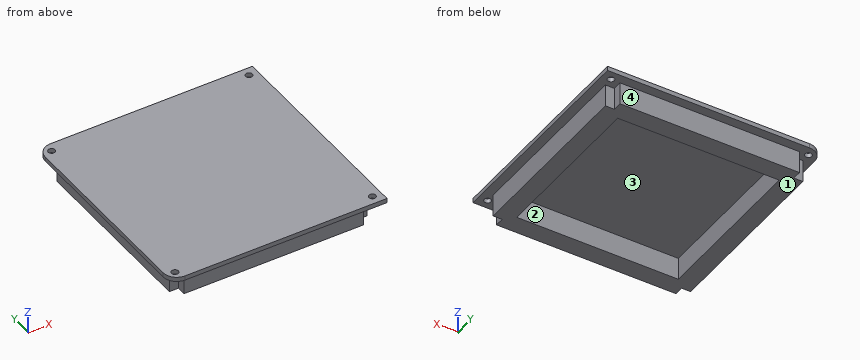
from build123d import *

# Parameters (mm, degrees)
F0_W     = 48
F0_H     = 48
F1_DEPTH = 1
F2_W     = 2
F2_H     = 2
F3_DEPTH = 5
F5_D     = 1.5
F6_R     = 3


with BuildPart() as f1:
    # F0 (on Top) → F1 (new body)
    with BuildSketch(Plane.XY):
        with Locations((-0.8524587825, -1.0040983325)):
            Rectangle(F0_W, F0_H)
        Polygon((19.1475412175, 18.9959016675), (21.1475412175, 18.9959016675), (21.1475412175, -21.0040983325), (19.1475412175, -21.0040983325), (19.1475412175, -23.0040983325), (-20.8524587825, -23.0040983325), (-20.8524587825, -21.0040983325), (-22.8524587825, -21.0040983325), (-22.8524587825, 18.9959016675), (-20.8524587825, 18.9959016675), (-20.8524587825, 20.9959016675), (19.1475412175, 20.9959016675), align=None, mode=Mode.SUBTRACT)
        Polygon((21.1475412175, -21.0040983325), (21.1475412175, 18.9959016675), (19.1475412175, 18.9959016675), (19.1475412175, 20.9959016675), (-20.8524587825, 20.9959016675), (-20.8524587825, 18.9959016675), (-22.8524587825, 18.9959016675), (-22.8524587825, -21.0040983325), (-20.8524587825, -21.0040983325), (-20.8524587825, -23.0040983325), (19.1475412175, -23.0040983325), (19.1475412175, -21.0040983325), align=None)
    extrude(amount=F1_DEPTH)

    # F2 (on Top) → F3 (join)
    with BuildSketch(Plane.XY):
        Polygon((-20.8524587825, -21.0040983325), (-20.8524587825, -23.0040983325), (19.1475412175, -23.0040983325), (19.1475412175, -21.0040983325), (17.1475412175, -21.0040983325), (17.1475412175, -19.0040983325), (-18.8524587825, -19.0040983325), (-18.8524587825, -21.0040983325), align=None)
        Polygon((-22.8524587825, -21.0040983325), (-20.8524587825, -21.0040983325), (-20.8524587825, -19.0040983325), (-18.8524587825, -19.0040983325), (-18.8524587825, 16.9959016675), (-20.8524587825, 16.9959016675), (-20.8524587825, 18.9959016675), (-22.8524587825, 18.9959016675), align=None)
        with Locations((-19.8524587825, -20.0040983325)):
            Rectangle(F2_W, F2_H)
        with Locations((18.1475412175, -20.0040983325)):
            Rectangle(F2_W, F2_H)
        Polygon((19.1475412175, -19.0040983325), (19.1475412175, -21.0040983325), (21.1475412175, -21.0040983325), (21.1475412175, 18.9959016675), (19.1475412175, 18.9959016675), (19.1475412175, 16.9959016675), (17.1475412175, 16.9959016675), (17.1475412175, -19.0040983325), align=None)
        with Locations((-19.8524587825, 17.9959016675)):
            Rectangle(F2_W, F2_H)
        Polygon((-18.8524587825, 18.9959016675), (-18.8524587825, 16.9959016675), (17.1475412175, 16.9959016675), (17.1475412175, 18.9959016675), (19.1475412175, 18.9959016675), (19.1475412175, 20.9959016675), (-20.8524587825, 20.9959016675), (-20.8524587825, 18.9959016675), align=None)
        with Locations((18.1475412175, 17.9959016675)):
            Rectangle(F2_W, F2_H)
    extrude(amount=-F3_DEPTH)

    # F5 (through all)
    with Locations(Plane.XY.offset(1)):
        with Locations((-22.8524587825, 20.9959016675), (-22.8524587825, -23.0040983325), (21.1475412175, -23.0040983325), (21.1475412175, 20.9959016675)):
            Hole(F5_D / 2)

    # F6
    f6_edges = [f1.edges().sort_by_distance(p)[0] for p in [
        (-24.852459, -25.004098, 0.5),
        (-24.852459, 22.995902, 0.5),
    ]]
    fillet(f6_edges, radius=F6_R)


solid = f1.part
Design review of the part built by this model. Coordinates are the model's own, in mm. Face numbers are marked on the shaded views. A direction names the side the tool comes from. Coordinates: 2 decimals unless noted, no trailing zeros. Loops run counter-clockwise (first coordinate to the right, second up) from the corner with the lowest first, then second, coordinate; pieces in that order, holes last. Notation, with made-up numbers: (-5.5, 61) -> (36.5, 61) arc R28 ccw to (36.5, 92) -> close; hole circle Ø5 at (6, -17). An arc over 180 degrees is marked (long way). Use a Markdown table: item, result. Add a question column.
Item 1: We need section A-A, the plane z = -1.3. Write out the cut boundary in (x, y).
Item 2: Machinability: for the marked faces 1 and 2, which of the approach directions +Z, -Z, +X, -X, +Y, -Y give a long, thin tool a straight path to every point of the face, cutting with its end or side? Answer none if there is none.
Item 3: We need section C-C, the plane y = -16. Write out the cut boundary in (x, z), and give its area (3 significant figures).
Item 4: We need section B-B, the plane x = 16. Write out the cut boundary in (y, z), and give its area (3 significant figures).
Item 5: The part is to be moulded in two halves that separate along X. For the marked faces 3 and 4, say which applies: +X half, -X half, draft (parallel to the pull), parting line (faces both ways), or undercut.
Item 6: Clearance check with flat-ended pins moving along their axes: P1, Ø2, axis at x = 20.5, z = -1.5, coming from the +Y side; P2, Ø1.6, axis at x = -21.5, z = -2, coming from the +Y side; P3, Ø2.5, axis at y = 1.5, z = -2.5, coming from the +X side. State where each tip first meets the part, or that it passes through.
Item 7: Wall thickness on L1, parallel to X at y = -1.5, z = -1.15; L2, parallel to Y at x = 6.5, z = -0.9; L3, parallel to Z at x = 15, y = 10.5: over which ranges is each line inside the solid? List them lowest first. Write a range as from..to.
Numbers:
| question | item | result |
|---|---|---|
| 1 | outline | (-22.85, -21) -> (-20.85, -21) -> (-20.85, -23) -> (19.15, -23) -> (19.15, -21) -> (21.15, -21) -> (21.15, 19) -> (19.15, 19) -> (19.15, 21) -> (-20.85, 21) -> (-20.85, 19) -> (-22.85, 19) -> close; hole (-18.85, -19) -> (17.15, -19) -> (17.15, 17) -> (-18.85, 17) -> close |
| 2 | face 1 | -Z, +X, -X, +Y, -Y |
| 2 | face 2 | -Z |
| 3 | outline | (-24.85, 0) -> (-22.85, 0) -> (-22.85, -5) -> (-18.85, -5) -> (-18.85, 0) -> (17.15, 0) -> (17.15, -5) -> (21.15, -5) -> (21.15, 0) -> (23.15, 0) -> (23.15, 1) -> (-24.85, 1) -> close |
| 3 | area | 88.0 mm^2 |
| 4 | outline | (-25, 0) -> (-23, 0) -> (-23, -5) -> (-19, -5) -> (-19, 0) -> (17, 0) -> (17, -5) -> (21, -5) -> (21, 0) -> (23, 0) -> (23, 1) -> (-25, 1) -> close |
| 4 | area | 88.0 mm^2 |
| 5 | face 3 | undercut |
| 5 | face 4 | draft |
| 6 | P1 | stops at y = 19 |
| 6 | P2 | stops at y = 21 |
| 6 | P3 | stops at x = 21.15 |
| 7 | L1 | x = -22.85..-18.85, 17.15..21.15 |
| 7 | L2 | y = -23..-19, 17..21 |
| 7 | L3 | z = 0..1 |
